Check sheet for the modelled part. Datum: model origin and axes. Units: mm. Face numbers are marked on the shaded views. A direction names the side the tool comes from. Round coordinates to 2 decimals unless told otherwise and drop trailing zeros. Order: outer loops, then holes, each group sorted by start corner. A loop starts at its lowest first (then second) coordinate and runs counter-clockwise, first axis right, second up. Notation, with made-up numbers: M 71.5,17 L 76.5,17 A22 cw 76.5,24 Z; hole C -34,-33 d8. An arc over 180 degrees is marked long. One line per item, written item: value. Start each with the question number.
(1) Release check for a two-part mould opening along Z. For the marked faces 1, 2 and 3 record: released by +Z, released by -Z, zero draft, split by the parting line, or undercut.
(2) Thickness scan on L1, parallel to Z at x = 2, y = 0; L2, parallel to Z at x = 20, y = 0; L3, parallel to Z at x = 63, y = -2.5. Record the ranges inside material, lowest first.
(3) Depth check by flat-ended pin: pin 1 Ø5.5 at (y, z) = (-33, 0) entering from +X; pin 2 Ø4.5 at (y, z) = (33, 0) entering from +X; pin 3 Ø12 at (x, y) = (25.5, -30.5) entering from +Z. Enter the tip coordinate at first touch or a pass-through.
(4) Access from +Z, -Z, +X, -X, +Y, -Y to the whole of each face (thin tool, end or side, straight path). Record for the marked faces 4, 5 and 6.
(5) Cross-section at B-B, the plane x = 30.5. Enter the section's corners in (y, z).
(6) Cross-section at A-A, the plane x = 16. Enter the section's corners in (y, z), and give its area (3 significant figures).
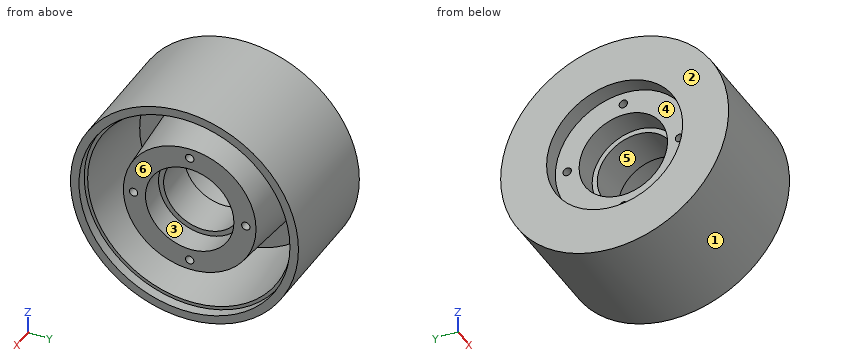
Autodesk Inventor part; units mm, degrees
ref_plane "YZ Plane" through (0, 0, 0) normal (1, 0, 0) x (0, 1, 0)
ref_plane "XZ Plane" through (0, 0, 0) normal (0, 1, 0) x (-1, 0, 0)
ref_plane "XY Plane" through (0, 0, 0) normal (0, 0, 1) x (1, 0, 0)
sketch "Boceto1" plane through (0, 0, 0) normal (0, 0, 1) x (1, 0, 0)
  line L0 (0, 0) -> (0, 40)
  line L1 (0, 40) -> (10, 40)
  line L2 (0, 0) -> (80, 0)
  line L3 (10, 40) -> (10, 0)
  line L4 (10, 0) -> (10, 26)
  line L5 (10, 26) -> (25, 26)
  line L6 (25, 26) -> (25, 0)
  line L7 (25, 0) -> (25, 23)
  line L8 (0, 0) -> (0, 67)
  line L9 (0, 67) -> (70, 67)
  line L10 (0, 67) -> (12, 67) construction
  line L11 (12, 67) -> (12, 0) construction
  line L12 (70, 67) -> (70, 62)
  line L13 (70, 62) -> (64, 62)
  line L14 (70, 62) -> (70, 0)
  line L15 (64, 0) -> (70, 0)
  line L16 (64, 0) -> (70, 0)
  line L17 (64, 62) -> (64, 0)
  line L18 (64, 62) -> (64, 60)
  line L19 (64, 0) -> (64, 39)
  line L20 (64, 60) -> (116.3905, 60) construction
  line L21 (64, 39) -> (116.3905, 39) construction
  line L22 (25, 0) -> (25, 23)
  line L23 (49, 0) -> (49, 23)
  line L24 (49, 23) -> (25, 23)
  line L25 (49, 23) -> (49, 26)
  line L26 (49, 26) -> (64, 26)
  line L27 (64, 39) -> (64, 49.5)
  line L28 (64, 49.5) -> (-5.756, 49.5) construction
  line L29 (12, 49.5) -> (12, 56)
  line L30 (12, 56) -> (12, 43)
  line L31 (12, 56) -> (64, 60)
  line L32 (64, 39) -> (12, 43)
  dimension "d0" = 40
  dimension "d1" = 10
  dimension "d2" = 80
  dimension "d3" = 26
  dimension "d4" = 15
  dimension "d10" = 67
  dimension "d12" = 70
  dimension "d16" = 12
  dimension "d22" = 5
  dimension "d29" = 54
  dimension "d30" = 2
  dimension "d31" = 39
  dimension "d40" = 24
  dimension "d41" = 23
  dimension "d42" = 3
  dimension "d45" = 10.5
  dimension "d46" = 6.5
  dimension "d47" = 13
revolve "Revolución1" add sketch "Boceto1" angle 360 about axis through (0, 0, 0) along (1, 0, 0) contours L8 L9 L12 L13 L17 L31 L29 L30 L32 L26 L25 L24 L6 L5 L3 L1
sketch "Boceto4" plane through (10, 0, 0) normal (-1, 0, 0) x (0, 0, 1)
  circle A0 centre (0, 0) radius 33 construction
  circle A1 centre (0, 0) radius 33 construction
  circle A2 centre (0, 0) radius 33 construction
  circle A3 centre (0, 0) radius 33 construction
  point P0 (-33, 0)
  point P1 (0, -33)
  point P2 (33, 0)
  point P3 (0, 33)
  dimension "d61" = 66
  dimension "d64" = 360
hole "Agujero2" at (10, 33, 0) at (10, 0, 33) at (10, -33, 0) at (10, 0, -33) direction (1, 0, 0) diameter 4.917 depth 15 tip angle 118
sketch "Boceto5" plane through (64, 0, 0) normal (1, 0, 0) x (0, 0, -1)
  circle A0 centre (0, 0) radius 33 construction
  circle A1 centre (0, 33) radius 2.4585
  circle A2 centre (-33, 0) radius 2.4585
  circle A3 centre (33, 0) radius 2.4585
  circle A4 centre (0, -33) radius 2.4585
  dimension "d73" = 66
hole "Agujero3" at (64, 33, 0) at (64, 0, 33) at (64, 0, -33) at (64, -33, 0) direction (-1, 0, 0) diameter 4.917 depth 18 tip angle 118
properties part number "Cilindro Tensor"
Values found:
1. face 1: split by the parting line
1. face 2: zero draft
1. face 3: undercut
2. L1: -67 to -40, 40 to 67
2. L2: -67 to -56.62, -42.38 to -35.46, -30.54 to -26, 26 to 30.54, 35.46 to 42.38, 56.62 to 67
2. L3: -66.95 to -59.87, -39 to -25.88, 25.88 to 39, 59.87 to 66.95
3. pin 1: x = 64
3. pin 2: x = 45.87
3. pin 3: z = 62.36
4. face 4: -X
4. face 5: +X, -X
4. face 6: +X
5. outline: C 0,0 d134; C 0,0 d83.15; hole C 0,0 d114.85; hole C 0,0 d46
6. outline: C 0,0 d134; C 0,0 d85.38; hole C 0,0 d112.62; hole C -33,0 d4.92; hole C 0,0 d52; hole C 0,-33 d4.92; hole C 0,33 d4.92; hole C 33,0 d4.92
6. area: 7,670 mm^2
